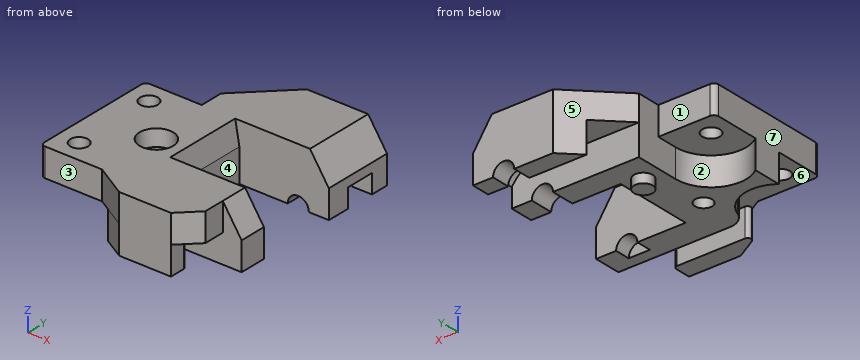
```python
from build123d import *

# Parameters (mm, degrees)
BOSS_EXTRUDE1_DEPTH                            = 6
BOSS_EXTRUDE3_DEPTH                            = 6
CBORE_FOR_6_SOCKET_HEAD_CAP_SCREW1_D           = 3.6576
CBORE_FOR_6_SOCKET_HEAD_CAP_SCREW1_CBORE_D     = 7.14502
CBORE_FOR_6_SOCKET_HEAD_CAP_SCREW1_CBORE_DEPTH = 3.5052
F_6_CLEARANCE_HOLE1_D                          = 3.7973
F_6_CLEARANCE_HOLE1_DEPTH                      = 17.47
F_6_CLEARANCE_HOLE1_TIP                        = 1.140824014
BOSS_EXTRUDE5_DEPTH                            = 15
BOSS_EXTRUDE6_DEPTH                            = 5.75
CUT_EXTRUDE1_START                             = -20
SKETCH11_5_R                                   = 2.25
CUT_EXTRUDE1_DEPTH                             = 35
CUT_EXTRUDE2_DEPTH                             = 6.1
CHAMFER2_SIZE                                  = 10
SKETCH26_R                                     = 2
BOSS_EXTRUDE10_DEPTH                           = 2
CHAMFER3_SIZE                                  = 5
CHAMFER3_SIZE2                                 = 0.881634904
BOSS_EXTRUDE7_DEPTH                            = 6
BOSS_EXTRUDE9_DEPTH                            = 6


with BuildPart() as part:
    # Sketch2 → Boss-Extrude1 (new body)
    with BuildSketch(Plane.XY):
        with BuildLine():
            Line((1, 0), (20, 0))
            Line((20, 0), (20, 27))
            Line((20, 27), (1, 27))
            ThreePointArc((1, 27), (0.292893219, 26.707106781), (0, 26))
            Line((0, 26), (0, 1))
            ThreePointArc((0, 1), (0.292893219, 0.292893219), (1, 0))
        make_face()
    extrude(amount=BOSS_EXTRUDE1_DEPTH)

    # Sketch3 → Boss-Extrude3 (add)
    with BuildSketch(Plane.XY):
        with BuildLine():
            ThreePointArc((0, 10.5), (6.616034902, 11.695303767), (11.531693039, 7.108695652))
            ThreePointArc((11.531693039, 7.108695652), (12.997768364, 5.216311724), (15.281929326, 4.5))
            Line((15.281929326, 4.5), (20, 4.5))
            Line((20, 4.5), (20, 27))
            Line((20, 27), (12, 27))
            Line((12, 27), (12, 22.5))
            ThreePointArc((12, 22.5), (7.854101966, 15.791796068), (0, 16.5))
            Line((0, 16.5), (0, 10.5))
        make_face()
    extrude(amount=-BOSS_EXTRUDE3_DEPTH)

    # CBORE for #6 Socket Head Cap Screw1 (through all)
    with Locations(Plane.XY.offset(6)):
        with Locations((13.5, 13.5)):
            CounterBoreHole(CBORE_FOR_6_SOCKET_HEAD_CAP_SCREW1_D / 2, CBORE_FOR_6_SOCKET_HEAD_CAP_SCREW1_CBORE_D / 2, CBORE_FOR_6_SOCKET_HEAD_CAP_SCREW1_CBORE_DEPTH)

    # #6 Clearance Hole1
    with Locations(Plane(origin=(0, 0, 0), x_dir=(-1, 0, 0), z_dir=(0, 0, -1))):
        with Locations((-4.5, 22.5), (-4.5, 4.5)):
            Hole(F_6_CLEARANCE_HOLE1_D / 2, depth=F_6_CLEARANCE_HOLE1_DEPTH)
            with Locations((0, 0, -(F_6_CLEARANCE_HOLE1_DEPTH + F_6_CLEARANCE_HOLE1_TIP / 2))):  # 118° drill point
                Cone(0, F_6_CLEARANCE_HOLE1_D / 2, F_6_CLEARANCE_HOLE1_TIP, mode=Mode.SUBTRACT)

    # Sketch11 → Boss-Extrude5 (add)
    with BuildSketch(Plane(origin=(0, 27, 0), x_dir=(1, 0, 0), z_dir=(0, 1, 0))):
        Polygon((12, 6), (12, -6), (35, -6), (39, 0), (39, 6), align=None)
    extrude(amount=BOSS_EXTRUDE5_DEPTH)

    # Sketch13 → Boss-Extrude6 (add)
    with BuildSketch(Plane(origin=(0, 10.25, 0), x_dir=(-1, 0, 0), z_dir=(0, -1, 0))):
        Polygon((-20, 6), (-39, 6), (-39, 0), (-35, -6), (-20, -6), align=None)
    extrude(amount=BOSS_EXTRUDE6_DEPTH)

    # Sketch11<5> → Cut-Extrude1 (cut)
    with BuildSketch(Plane(origin=(0, 27, 0), x_dir=(1, 0, 0), z_dir=(0, 1, 0)).offset(CUT_EXTRUDE1_START)):
        with Locations((32.5, 6)):
            Circle(SKETCH11_5_R)
    extrude(amount=CUT_EXTRUDE1_DEPTH, mode=Mode.SUBTRACT)

    # Sketch14 → Cut-Extrude2 (cut)
    with BuildSketch(Plane(origin=(0, 32, 0), x_dir=(-1, 0, 0), z_dir=(0, -1, 0))):
        with BuildLine():
            Line((-29.85, 12.55), (-29.85, -0.55))
            Line((-29.85, -0.55), (-28.547785431, -0.55))
            ThreePointArc((-28.547785431, -0.55), (-25.8382832, 2.239145141), (-24.85, 6))
            ThreePointArc((-24.85, 6), (-25.8382832, 9.760854859), (-28.547785431, 12.55))
            Line((-28.547785431, 12.55), (-29.85, 12.55))
        make_face()
        with BuildLine():
            Line((-28.547785431, -0.55), (-29.85, -0.55))
            Line((-29.85, -0.55), (-29.85, 12.55))
            Line((-29.85, 12.55), (-28.547785431, 12.55))
            ThreePointArc((-28.547785431, 12.55), (-40.15, 6), (-28.547785431, -0.55))
        make_face()
        with BuildLine():
            ThreePointArc((-24.85, 6), (-25.8382832, 2.239145141), (-28.547785431, -0.55))
            Line((-28.547785431, -0.55), (-24.85, -0.55))
            Line((-24.85, -0.55), (-24.85, 6))
        make_face()
        Polygon((-24.85, 6), (-24.85, -0.55), (-9.85, -0.55), (-9.85, 12.55), (-24.85, 12.55), align=None)
        with BuildLine():
            Line((-24.85, 12.55), (-28.547785431, 12.55))
            ThreePointArc((-28.547785431, 12.55), (-25.8382832, 9.760854859), (-24.85, 6))
            Line((-24.85, 6), (-24.85, 12.55))
        make_face()
    extrude(amount=-CUT_EXTRUDE2_DEPTH, mode=Mode.SUBTRACT)

    # Chamfer2
    chamfer2_edges = [part.edges().sort_by_distance(p)[0] for p in [
        (12, 42, 0),
    ]]
    chamfer(chamfer2_edges, length=CHAMFER2_SIZE)

    # Sketch26 → Boss-Extrude10 (add)
    with BuildSketch(Plane(origin=(0, 0, -6), x_dir=(-1, 0, 0), z_dir=(0, 0, -1))):
        with Locations((-16, 26)):
            Circle(SKETCH26_R)
    extrude(amount=BOSS_EXTRUDE10_DEPTH)

    # Chamfer3
    chamfer3_edges = [part.edges().sort_by_distance(p)[0] for p in [
        (20, 18.625, 6),
    ]]
    chamfer3_side = [part.faces().sort_by_distance(p)[0] for p in [
        (20, 18.625, 0),
    ]]
    chamfer(chamfer3_edges, length=CHAMFER3_SIZE, length2=CHAMFER3_SIZE2, reference=chamfer3_side[0])

    # Sketch15 → Boss-Extrude7 (add)
    with BuildSketch(Plane.XY.offset(6)):
        Polygon((20, 4.5), (20, 0), (13.07179677, 0), (20, -4), (31, -4), (35, 0), (35, 4.5), align=None)
    extrude(amount=-BOSS_EXTRUDE7_DEPTH)

    # Sketch17 → Boss-Extrude9 (add)
    with BuildSketch(Plane(origin=(0, 0, 0), x_dir=(-1, 0, 0), z_dir=(0, 0, -1))):
        with BuildLine():
            Line((-30.25, 0), (-15.870834875, 0))
            ThreePointArc((-15.870834875, 0), (-15.146390506, -0.555885716), (-15.495834875, -1.399519053))
            Line((-15.495834875, -1.399519053), (-20, -4))
            Line((-20, -4), (-31, -4))
            Line((-31, -4), (-31, -0.75))
            ThreePointArc((-31, -0.75), (-30.780330086, -0.219669914), (-30.25, 0))
        make_face()
    extrude(amount=BOSS_EXTRUDE9_DEPTH)


solid = part.part
```
Build history of the part. All positions in model axes, mm. Face numbers are marked on the shaded views. A direction names the side the tool comes from. Coordinates: 2 decimals unless noted, no trailing zeros. Order: outer loops, then holes, each group sorted by start corner. A loop starts at its lowest first (then second) coordinate and runs counter-clockwise, first axis right, second up.
Item 1: Saw through at D-D on y = 34. List the corners of the cut face in (x, z), then the cut area to 3 significant figures.
Filled in:
outline: (14, 0.55) - (28.55, 0.55) arc R7.65 cw to (39, -1.97) - (39, 0) - (35, 6) - (14, 6) - close
area: 121 mm2
Item 2: Mould opens along Y. For the marked faces 5, 6 and 7 say: released by +Y, released by -Y, zero draft, split by the parting line, or undercut.
Filled in:
face 5: released by +Y
face 6: undercut
face 7: zero draft
Item 3: Saw through at C-C on z = 5.25. List the corners of the cut face in (x, y).
Filled in:
outline: (0, 1) arc R1 ccw to (1, 0) - (13.07, 0) - (20, -4) - (31, -4) - (35, 0) - (35, 4.5) - (35.5, 4.5) - (35.5, 10.25) - (19.25, 10.25) - (19.25, 27) - (35.5, 27) - (35.5, 42) - (22, 42) - (12, 32) - (12, 27) - (1, 27) arc R1 ccw to (0, 26) - close; hole circle Ø3.8 at (4.5, 4.5); hole circle Ø3.8 at (4.5, 22.5); hole circle Ø7.15 at (13.5, 13.5)
Item 4: Drop flat-ended pins along their axis: pin 1 Ø4 at (y, z) = (24.5, -2.5) entering from +X; pin 2 Ø1.5 at (x, y) = (5, 4.5) entering from +Z; pin 3 Ø4 at (x, y) = (11.5, 1) entering from -Z; pin 4 Ø13 at (x, y) = (7.5, 22.5) entering from -Z. Give the stop position or say it passes through.
Filled in:
pin 1: stops at x = 20
pin 2: passes through
pin 3: stops at z = 0
pin 4: stops at z = -6
Item 5: Saw through at B-B on y = 29. List the corners of the cut face in (x, z), then the cut area to 3 significant figures.
Filled in:
outline: (12, -6) - (30.25, -6) arc R2.25 cw to (34.75, -6) - (39, -6) - (39, 0) - (35, 6) - (12, 6) - close
area: 304 mm2
Item 6: Tool access for the marked faces 1, 2, 3 and 4: list every direction of +Z, -Z, +X, -X, +Y, -Y with a clear straight run to the whole face (end or side of a thin tool).
Filled in:
face 1: +Z, -Z, -X, +Y
face 2: -Z, +Y
face 3: +Z, -Z, -X, -Y
face 4: +Z, -Z, +X
Item 7: Saw through at A-A on x = 33.5. List the corners of the cut face in (y, z).
Filled in:
outline: (-1.5, 0) - (4.5, 0) - (4.5, -6) - (7, -6) - (7, -3.98) - (10.25, -3.98) - (10.25, 6) - (-1.5, 6) - close; (27, -3.98) - (32, -3.98) - (32, 1.58) - (38.1, 1.58) - (38.1, -3.98) - (42, -3.98) - (42, 6) - (27, 6) - close
Item 8: Drill centre lines: L1, parallel to Z at x = 2, y = 1.5; L2, parallel to Z at x = 27, y = 9.5; L3, parallel to Y at x = 13.5, z = 5.2. Where is each one in solid material? Low to high.
Filled in:
L1: z = 0 to 6
L2: z = -6 to 6
L3: y = -0.25 to 9.93, 17.07 to 33.5
